Check sheet for the modelled part. Datum: model origin and axes. Units: mm. A direction names the side the tool comes from. Give positions to 0.01 mm unless a question says otherwise; leave off trailing zeros. Order: outer loops, then holes, each group sorted by start corner. A loop starts at its lowest first (then second) coordinate and runs counter-clockwise, first axis right, second up. Notation, with made-up numbers: (-4.5, 48.5) -> (9.5, 48.5) arc R23 cw to (9.5, 67.5) -> close; hole circle Ø7 at (70, 42). An arc over 180 degrees is marked (long way). Write each question's results on one line, items separated by ' | '.
from build123d import *

# Parameters (mm, degrees)
SKETCH_1_R          = 32.5
SKETCH_1_R_2        = 30
EXTRUDE_1_DEPTH     = 340
SKETCH_2_R          = 32.5
EXTRUDE_2_DEPTH     = 5
SKETCH_8_R          = 1.5
CUT_EXTRUDE_2_DEPTH = 5
SKETCH_9_R          = 32.5
SKETCH_9_R_2        = 30
EXTRUDE_3_DEPTH     = 260
SKETCH_10_R         = 32.5
EXTRUDE_4_DEPTH     = 2
CUT_EXTRUDE_3_DEPTH = 2
SKETCH_14_W         = 65
SKETCH_14_H         = 180
CUT_EXTRUDE_4_DEPTH = 32.5
FILLET_1_R          = 1


with BuildPart() as part:
    # 草图1 → 凸台-拉伸1 (new body)
    with BuildSketch(Plane(origin=(0, 0, 0), x_dir=(1, 0, 0), z_dir=(0, 1, 0))):
        with Locations(Location((0, 0, 0), (0, 0, 270))):
            Circle(SKETCH_1_R)
        with Locations(Location((0, 0, 0), (0, 0, 270))):
            Circle(SKETCH_1_R_2, mode=Mode.SUBTRACT)
    extrude(amount=EXTRUDE_1_DEPTH)

    # 草图2 → 凸台-拉伸2 (add)
    with BuildSketch(Plane(origin=(0, 340, 0), x_dir=(1, 0, 0), z_dir=(0, 1, 0))):
        with Locations(Location((0, 0, 0), (0, 0, 270))):
            Circle(SKETCH_2_R)
    extrude(amount=EXTRUDE_2_DEPTH)

    # 草图8 → 切除-拉伸2 (cut)
    with BuildSketch(Plane(origin=(0, 345, 0), x_dir=(1, 0, 0), z_dir=(0, 1, 0))):
        with Locations(Location((-13.1, 0, 0), (0, 0, 270))):
            Circle(SKETCH_8_R)
        with Locations(Location((13.1, 0, 0), (0, 0, 270))):
            Circle(SKETCH_8_R)
        with BuildLine():
            Line((10.3, -10.1), (10.3, 10.1))
            ThreePointArc((10.3, 10.1), (9.854035247, 11.427915792), (8.696945136, 12.217464641))
            ThreePointArc((8.696945136, 12.217464641), (8.401311956, 12.279268479), (8.1, 12.3))
            Line((8.1, 12.3), (-8.1, 12.3))
            ThreePointArc((-8.1, 12.3), (-8.401311956, 12.279268479), (-8.696945136, 12.217464641))
            ThreePointArc((-8.696945136, 12.217464641), (-9.854035247, 11.427915792), (-10.3, 10.1))
            Line((-10.3, 10.1), (-10.3, -10.1))
            ThreePointArc((-10.3, -10.1), (-9.854035247, -11.427915792), (-8.696945136, -12.217464641))
            ThreePointArc((-8.696945136, -12.217464641), (-8.401311956, -12.279268479), (-8.1, -12.3))
            Line((-8.1, -12.3), (8.1, -12.3))
            ThreePointArc((8.1, -12.3), (8.401311956, -12.279268479), (8.696945136, -12.217464641))
            ThreePointArc((8.696945136, -12.217464641), (9.854035247, -11.427915792), (10.3, -10.1))
        make_face()
    extrude(amount=-CUT_EXTRUDE_2_DEPTH, mode=Mode.SUBTRACT)

    # 草图9 → 凸台-拉伸3 (add)
    with BuildSketch(Plane(origin=(0, 345, 0), x_dir=(1, 0, 0), z_dir=(0, 1, 0))):
        with Locations(Location((0, 0, 0), (0, 0, 270))):
            Circle(SKETCH_9_R)
        with Locations(Location((0, 0, 0), (0, 0, 270))):
            Circle(SKETCH_9_R_2, mode=Mode.SUBTRACT)
    extrude(amount=EXTRUDE_3_DEPTH)

    # 草图10 → 凸台-拉伸4 (add)
    with BuildSketch(Plane(origin=(0, 605, 0), x_dir=(1, 0, 0), z_dir=(0, 1, 0))):
        with Locations(Location((0, 0, 0), (0, 0, 270))):
            Circle(SKETCH_10_R)
    extrude(amount=EXTRUDE_4_DEPTH)

    # 草图12 → 切除-拉伸3 (cut)
    with BuildSketch(Plane(origin=(0, 607, 0), x_dir=(1, 0, 0), z_dir=(0, 1, 0))):
        with BuildLine():
            ThreePointArc((12.95, 11.5), (11.5, 12.95), (10.05, 11.5))
            ThreePointArc((10.05, 11.5), (11.5, 10.05), (12.95, 11.5))
        make_face()
        with BuildLine():
            ThreePointArc((12.95, -11.5), (11.5, -10.05), (10.05, -11.5))
            ThreePointArc((10.05, -11.5), (11.5, -12.95), (12.95, -11.5))
        make_face()
        with BuildLine():
            ThreePointArc((11.2, 0), (0, 11.2), (-11.2, 0))
            ThreePointArc((-11.2, 0), (0, -11.2), (11.2, 0))
        make_face()
        with BuildLine():
            ThreePointArc((-10.05, -11.5), (-11.5, -10.05), (-12.95, -11.5))
            ThreePointArc((-12.95, -11.5), (-11.5, -12.95), (-10.05, -11.5))
        make_face()
        with BuildLine():
            ThreePointArc((-10.05, 11.5), (-11.5, 12.95), (-12.95, 11.5))
            ThreePointArc((-12.95, 11.5), (-11.5, 10.05), (-10.05, 11.5))
        make_face()
    extrude(amount=-CUT_EXTRUDE_3_DEPTH, mode=Mode.SUBTRACT)

    # 草图14 → 切除-拉伸4 (cut)
    with BuildSketch(Plane.XY):
        with Locations((0, 515)):
            Rectangle(SKETCH_14_W, SKETCH_14_H)
    extrude(amount=-CUT_EXTRUDE_4_DEPTH, mode=Mode.SUBTRACT)

    # 圆角1
    fillet_1_edges = [part.edges().sort_by_distance(p)[0] for p in [
        (0, 425, -32.5),
        (-30, 515, 0),
        (30, 515, 0),
        (-31.25, 605, 0),
        (-32.5, 515, 0),
        (-31.25, 425, 0),
        (0, 605, -32.5),
        (31.25, 425, 0),
        (32.5, 515, 0),
        (31.25, 605, 0),
        (21.213203436, 605, 21.213203436),
        (0, 425, -30),
    ]]
    fillet(fillet_1_edges, radius=FILLET_1_R)


solid = part.part
1. Section check A-A on y = 494.5. Record the cut outline in (x, z).
Verdict:
outline: (-32.48, 1.03) arc R1 ccw to (-31.48, 0) -> (-30.98, 0) arc R1 ccw to (-29.98, 0.97) arc R30 cw to (29.98, 0.97) arc R1 ccw to (30.98, 0) -> (31.48, 0) arc R1 ccw to (32.48, 1.03) arc R32.5 ccw to start
2. Gauge pin test, flat ends, axial feed: pin 1 Ø6 at (x, y) = (14.5, 368) entering from +Z; pin 2 Ø0.6 at (x, y) = (-31, 559.5) entering from -Z; pin 3 Ø3 at (x, z) = (22.5, 12.5) entering from -Y. Record the tip position at first contact, or that the pin passes through.
Verdict:
pin 1: stops at z = 30.4 | pin 2: stops at z = 0 | pin 3: stops at y = 340
3. Material ranges on probe 1 along Z at (x, y) = (0, 606.45); probe 2 along X at (y, z) = (212, 0); probe 3 along Y at (x, z) = (10.5, 5), recorded low to high. Write a range as from..to.
Verdict:
probe 1: z = -32.5..-11.2, 11.2..32.5 | probe 2: x = -32.5..-30, 30..32.5 | probe 3: y = 340..345, 605..607
4. Section check B-B on y = 315. Record the cut outline in (x, z).
Verdict:
outline: circle Ø65 at (0, 0); hole circle Ø60 at (0, 0)
5. Mould release check, pull along Y, two halves, no side actions. Record for faces 1 (the cylindrical face through (1.32, 167.62, -29.97)), 2 (the flat face through (-4.8, 425, -30.9)), 3 (the flat face through (0, 340, 13)): +Y half, -Y half, draft (parallel to the pull), parting line (faces both ways), or undercut.
Verdict:
face 1: draft | face 2: undercut | face 3: -Y half
6. Access from +Z, -Z, +X, -X, +Y, -Y to the whole of each face (thin tool, end or side, straight path). Record for faces 4 (the flat face through (0, 605, -14)), 5 (the cylindrical face through (9.76, 231.81, 31)), 6 (the flat face through (0, 345, 13)), 7 (the cylindrical face through (8.255, 606.014, 7.569)).
Verdict:
face 4: -Z | face 5: +Y, -Y | face 6: none | face 7: +Y
